```python
from build123d import *

# Parameters (mm, degrees)
BOSS_EXTRU_1_DEPTH      = 3
ESQUISSE2_R             = 1.75
ESQUISSE2_R_2           = 3.25
BOSS_EXTRU_2_DEPTH      = 5
ESQUISSE3_R             = 1
ESQUISSE3_R_2           = 2.5
ENL_V_MAT_EXTRU_1_DEPTH = 2.5


with BuildPart() as part:
    # Esquisse1 → Boss.-Extru.1 (new body)
    with BuildSketch(Plane(origin=(0, 0, 0), x_dir=(1, 0, 0), z_dir=(0, 1, 0))):
        with BuildLine():
            Line((10.2, -11.9), (-10.2, -11.9))
            ThreePointArc((-10.2, -11.9), (-22.1, 0), (-10.2, 11.9))
            Line((-10.2, 11.9), (10.2, 11.9))
            ThreePointArc((10.2, 11.9), (22.1, 0), (10.2, -11.9))
        make_face()
    extrude(amount=BOSS_EXTRU_1_DEPTH)

    # Esquisse2 → Boss.-Extru.2 (add)
    with BuildSketch(Plane(origin=(0, 3, 0), x_dir=(1, 0, 0), z_dir=(0, 1, 0))):
        with Locations(Location((-10.2, 0, 0), (0, 0, 270))):
            Circle(ESQUISSE2_R)
        with Locations(Location((10.2, 0, 0), (0, 0, 270))):
            Circle(ESQUISSE2_R_2)
    extrude(amount=BOSS_EXTRU_2_DEPTH)

    # Esquisse3 → Enlèv. mat.-Extru.1 (cut)
    with BuildSketch(Plane(origin=(0, 8, 0), x_dir=(1, 0, 0), z_dir=(0, 1, 0))):
        with Locations(Location((-10.2, 0, 0), (0, 0, 270))):
            Circle(ESQUISSE3_R)
        with Locations(Location((10.2, 0, 0), (0, 0, 270))):
            Circle(ESQUISSE3_R_2)
    extrude(amount=-ENL_V_MAT_EXTRU_1_DEPTH, mode=Mode.SUBTRACT)


solid = part.part
```
Verification items for the finished model (mm, model axes). A direction names the side the tool comes from. Coordinates: 2 decimals unless noted, no trailing zeros. Loops run counter-clockwise (first coordinate to the right, second up) from the corner with the lowest first, then second, coordinate; pieces in that order, holes last. Notation, with made-up numbers: (34.25, 42) -> (51.25, 42) arc R24 ccw to (51.25, 75) -> close; hole circle Ø9 at (72, 20.25). An arc over 180 degrees is marked (long way). Answer in a Markdown table with one row per item.
1) Section check D-D (y = 2.25). Record the cut outline in (x, z).
The answers:
| item | result |
|---|---|
| outline | (-10.2, -11.9) -> (10.2, -11.9) arc R11.9 ccw to (10.2, 11.9) -> (-10.2, 11.9) arc R11.9 ccw to start |
2) Section check C-C (x = -3). Record the cut outline in (y, z).
The answers:
| item | result |
|---|---|
| outline | (0, -11.9) -> (3, -11.9) -> (3, 11.9) -> (0, 11.9) -> close |
3) Scan lines: line 1 along X through (y, z) = (6.4, 0); line 2 along Y through (x, z) = (-0.5, 8); line 3 along Z through (x, y) = (-10, 4.5). Record each from-to range of solid material in increasing order. Write a range as from..to.
The answers:
| item | result |
|---|---|
| line 1 | x = -11.95..-11.2, -9.2..-8.45, 6.95..7.7, 12.7..13.45 |
| line 2 | y = 0..3 |
| line 3 | z = -1.74..1.74 |
4) Depth check by flat-ended pin: P1, Ø2, axis at x = -13.5, z = -0.5, coming from the +Y side; P2, Ø1, axis at y = 4.5, z = -6, coming from the +X side (3 decimals); P3, Ø1, axis at y = 5.5, z = 3, coming from the +X side; P4, Ø4, axis at x = 10.2, z = 0, coming from the +Y side. Enter the tip coordinate at first touch or a pass-through.
The answers:
| item | result |
|---|---|
| P1 | stops at y = 3 |
| P2 | passes through |
| P3 | stops at x = 12.28 |
| P4 | stops at y = 5.5 |
5) Access from +Z, -Z, +X, -X, +Y, -Y to the whole of each face (thin tool, end or side, straight path). Record for faces 1 (the face through (-8.465, 5.465, -0.228)), 2 (the face through (-22.097, 1.479, 0.262)).
The answers:
| item | result |
|---|---|
| face 1 | +Y |
| face 2 | -X, +Y, -Y |
6) Draft check along Z on faces 3 (the face through (0, 3, 0)), 4 (the face through (22.097, 1.479, -0.262)), 5 (the face through (10, 5.5, 0)). Enter one of: released by +Z, released by -Z, zero draft, split by the parting line, or undercut.
The answers:
| item | result |
|---|---|
| face 3 | zero draft |
| face 4 | split by the parting line |
| face 5 | undercut |
7) Section check A-A (y = 6.75). Record the cut outline in (x, z), and give its area (3 significant figures).
The answers:
| item | result |
|---|---|
| outline | circle Ø3.5 at (-10.2, 0); circle Ø6.5 at (10.2, 0); hole circle Ø2 at (-10.2, 0); hole circle Ø5 at (10.2, 0) |
| area | 20.0 mm2 |
8) Section check B-B (z = 0). Record the cut outline in (x, y).
The answers:
| item | result |
|---|---|
| outline | (-22.1, 0) -> (22.1, 0) -> (22.1, 3) -> (13.45, 3) -> (13.45, 8) -> (12.7, 8) -> (12.7, 5.5) -> (7.7, 5.5) -> (7.7, 8) -> (6.95, 8) -> (6.95, 3) -> (-8.45, 3) -> (-8.45, 8) -> (-9.2, 8) -> (-9.2, 5.5) -> (-11.2, 5.5) -> (-11.2, 8) -> (-11.95, 8) -> (-11.95, 3) -> (-22.1, 3) -> close |
